Geometry check sheet. Reference: drawing and pictorial views, mm from the part's lowest x, y, z. A direction names the side the tool comes from. Round coordinates to 2 decimals unless told otherwise and drop trailing zeros. Loops run counter-clockwise (first coordinate to the right, second up) from the corner with the lowest first, then second, coordinate; pieces in that order, holes last. Notation, with made-up numbers: (24, 17.25) -> (43, 17.25) arc R12 ccw to (43, 25.25) -> close; hole circle Ø1 at (-20, 10). An arc over 180 degrees is marked (long way). Use one line per item in the form item = value.
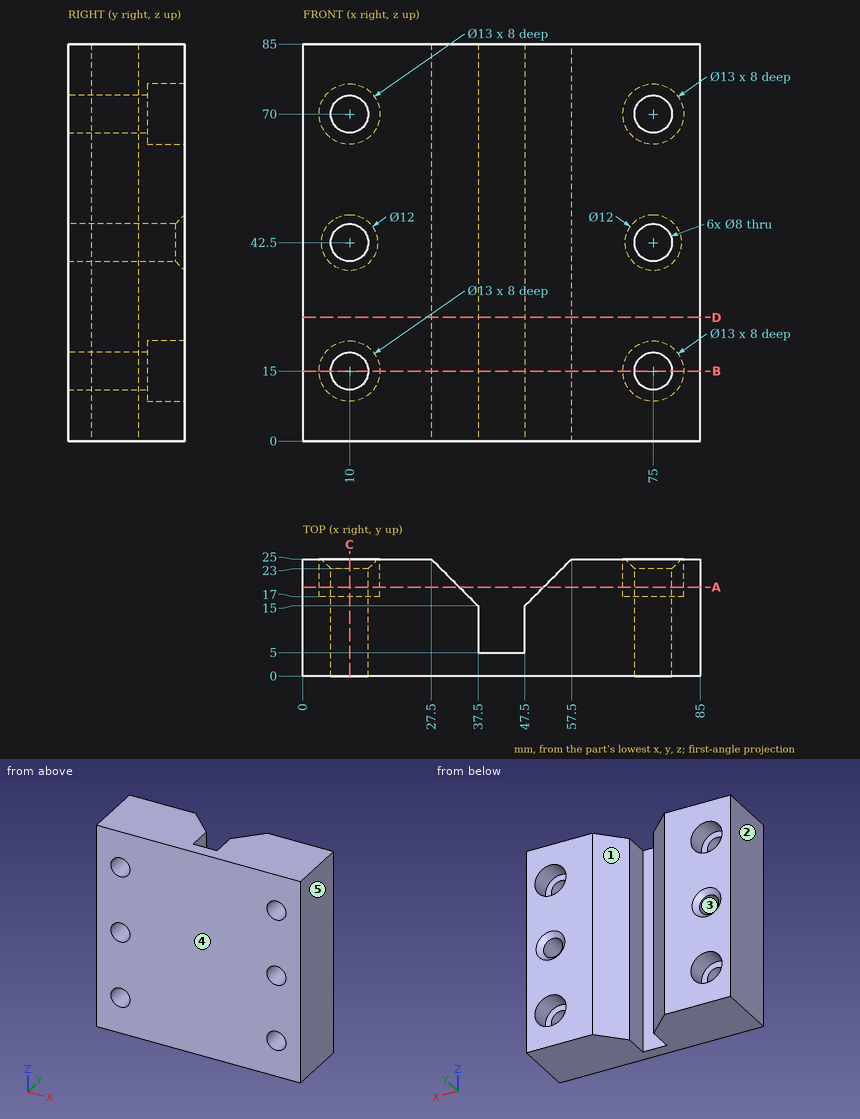
1. Section check C-C (x = 10). Record the boundary of the cut face in (y, z), then the cut area to 3 significant figures.
Return value:
outline = (0, 0) -> (25, 0) -> (25, 8.5) -> (17, 8.5) -> (17, 11) -> (0, 11) -> close; (0, 19) -> (17, 19) -> (17, 21.5) -> (25, 21.5) -> (25, 36.5) -> (23, 38.5) -> (0, 38.5) -> close; (0, 46.5) -> (23, 46.5) -> (25, 48.5) -> (25, 63.5) -> (17, 63.5) -> (17, 66) -> (0, 66) -> close; (0, 74) -> (17, 74) -> (17, 76.5) -> (25, 76.5) -> (25, 85) -> (0, 85) -> close
area = 1,440 mm2
2. Section check B-B (z = 15). Record the boundary of the cut face in (x, y).
Return value:
outline = (0, 0) -> (6, 0) -> (6, 17) -> (3.5, 17) -> (3.5, 25) -> (0, 25) -> close; (14, 0) -> (71, 0) -> (71, 17) -> (68.5, 17) -> (68.5, 25) -> (57.5, 25) -> (47.5, 15) -> (47.5, 5) -> (37.5, 5) -> (37.5, 15) -> (27.5, 25) -> (16.5, 25) -> (16.5, 17) -> (14, 17) -> close; (79, 0) -> (85, 0) -> (85, 25) -> (81.5, 25) -> (81.5, 17) -> (79, 17) -> close
3. Mould release check, pull along X, two halves, no side actions. Record for the marked faces 3, 4 and 5: released by +X, released by -X, zero draft, split by the parting line, or undercut.
Return value:
face_3 = undercut
face_4 = zero draft
face_5 = released by +X
4. Tool access check on the marked faces 1 and 2. Record the directions out of +Z, -Z, +X, -X, +Y, -Y that give a thin tool (end or side, any length) a straight path to the whole face; none if there is none.
Return value:
face_1 = +Z, -Z, +Y
face_2 = +Z, -Z, -X, +Y, -Y
5. Gauge pin test, flat ends, axial feed: pin 1 (10.5 mm diameter, centred on x = 10, z = 15, fed in from +Y); pin 2 (3 mm diameter, centred on x = 40.5, z = 25, fed in from +Y). Record the tip position at first contact, or that the pin passes through.
Return value:
pin_1 = 17
pin_2 = 5
6. Section check D-D (z = 26.5). Record the boundary of the cut face in (x, y).
Return value:
outline = (0, 0) -> (85, 0) -> (85, 25) -> (57.5, 25) -> (47.5, 15) -> (47.5, 5) -> (37.5, 5) -> (37.5, 15) -> (27.5, 25) -> (0, 25) -> close
7. Section check A-A (y = 19). Record the boundary of the cut face in (x, z).
Return value:
outline = (0, 0) -> (33.5, 0) -> (33.5, 85) -> (0, 85) -> close; (51.5, 0) -> (85, 0) -> (85, 85) -> (51.5, 85) -> close; hole circle Ø13 at (10, 15); hole circle Ø13 at (10, 70); hole circle Ø8 at (10, 42.5); hole circle Ø13 at (75, 15); hole circle Ø13 at (75, 70); hole circle Ø8 at (75, 42.5)
8. Material ranges on line 1 along X through (y, z) = (11.5, 15); line 2 along X through (y, z) = (8.5, 28); line 3 along X through (y, z) = (3, 69.5), recorded low to high.
Return value:
line_1 = 0 to 6, 14 to 37.5, 47.5 to 71, 79 to 85
line_2 = 0 to 37.5, 47.5 to 85
line_3 = 0 to 6.03, 13.97 to 71.03, 78.97 to 85
